```python
from build123d import *

# Parameters (mm, degrees)
SKETCH1_W               = 101.6
SKETCH1_H               = 203.2
BOSS_EXTRUDE1_DEPTH     = 101.6
SKETCH2_W               = 12.7
SKETCH2_H               = 12.7
SKETCH2_W_2             = 12.648057186
CUT_EXTRUDE1_DEPTH      = 203.2
SKETCH3_W               = 4.23418
SKETCH3_H               = 63.5
SKETCH3_W_2             = 63.551942814
SKETCH3_H_2             = 4.23418
SKETCH3_W_3             = 4.181475186
SKETCH3_W_4             = 8.466582
SKETCH3_H_3             = 8.46582
SKETCH3_W_5             = 8.46582
CUT_EXTRUDE2_DEPTH      = 200.025
SKETCH4_W               = 101.6
SKETCH4_H               = 25.341987408
CUT_EXTRUDE3_DEPTH      = 101.6
F_1_2_13_TAPPED_HOLE2_D = 10.71626
SKETCH7_W               = 13.255770889
SKETCH7_H               = 13.293622463
SKETCH7_W_2             = 13.104364594
SKETCH7_H_2             = 13.217919315
CUT_EXTRUDE4_DEPTH      = 190.5


with BuildPart() as part:
    # Sketch1 → Boss-Extrude1 (new body)
    with BuildSketch(Plane(origin=(0, 0, 0), x_dir=(0, 0, -1), z_dir=(1, 0, 0))):
        Rectangle(SKETCH1_W, SKETCH1_H)
    extrude(amount=BOSS_EXTRUDE1_DEPTH)

    # Sketch2 → Cut-Extrude1 (cut)
    with BuildSketch(Plane(origin=(0, 101.6, 0), x_dir=(1, 0, 0), z_dir=(0, 1, 0))):
        with Locations((9.525, 41.275)):
            Rectangle(SKETCH2_W, SKETCH2_H)
        with Locations((9.525, -41.275)):
            Rectangle(SKETCH2_W, SKETCH2_H)
        with Locations((92.100971407, -41.275)):
            Rectangle(SKETCH2_W_2, SKETCH2_H)
        with Locations((92.100971407, 41.275)):
            Rectangle(SKETCH2_W_2, SKETCH2_H)
    extrude(amount=-CUT_EXTRUDE1_DEPTH, mode=Mode.SUBTRACT)

    # Sketch3 → Cut-Extrude2 (cut)
    with BuildSketch(Plane(origin=(0, 101.6, 0), x_dir=(1, 0, 0), z_dir=(0, 1, 0))):
        with Locations((16.93291, 0)):
            Rectangle(SKETCH3_W, SKETCH3_H)
        with Locations((50.825971407, 0)):
            Rectangle(SKETCH3_W_2, SKETCH3_H)
        with Locations((50.825971407, 33.86709)):
            Rectangle(SKETCH3_W_2, SKETCH3_H_2)
        with Locations((84.692680407, 0)):
            Rectangle(SKETCH3_W_3, SKETCH3_H)
        with Locations((94.191709, 0)):
            Rectangle(SKETCH3_W_4, SKETCH3_H)
        with Locations((50.825971407, 43.39209)):
            Rectangle(SKETCH3_W_2, SKETCH3_H_3)
        with Locations((7.40791, 0)):
            Rectangle(SKETCH3_W_5, SKETCH3_H)
        with Locations((50.825971407, -43.39209)):
            Rectangle(SKETCH3_W_2, SKETCH3_H_3)
        with Locations((50.825971407, -33.86709)):
            Rectangle(SKETCH3_W_2, SKETCH3_H_2)
    extrude(amount=-CUT_EXTRUDE2_DEPTH, mode=Mode.SUBTRACT)

    # Sketch4 → Cut-Extrude3 (cut)
    with BuildSketch(Plane(origin=(101.6, 0, 0), x_dir=(0, 0, -1), z_dir=(1, 0, 0))):
        with Locations((0, 88.929006296)):
            Rectangle(SKETCH4_W, SKETCH4_H)
    extrude(amount=-CUT_EXTRUDE3_DEPTH, mode=Mode.SUBTRACT)

    # 1/2-13 Tapped Hole2 (through all)
    with Locations(Plane(origin=(50.825971407, -98.425, 0), x_dir=(0, 0, 1), z_dir=(0, 1, 0))):
        with Locations((0, 0)):
            Hole(F_1_2_13_TAPPED_HOLE2_D / 2)

    # Sketch7 → Cut-Extrude4 (cut)
    with BuildSketch(Plane(origin=(0, 76.258012592, 0), x_dir=(1, 0, 0), z_dir=(0, 1, 0))):
        with Locations((9.802885445, 40.978188769)):
            Rectangle(SKETCH7_W, SKETCH7_H)
        with Locations((91.872817703, 40.978188769)):
            Rectangle(SKETCH7_W_2, SKETCH7_H)
        with Locations((91.872817703, -41.016040343)):
            Rectangle(SKETCH7_W_2, SKETCH7_H_2)
        with Locations((9.802885445, -41.016040343)):
            Rectangle(SKETCH7_W, SKETCH7_H_2)
    extrude(amount=-CUT_EXTRUDE4_DEPTH, mode=Mode.SUBTRACT)


solid = part.part
```
Build history of the part. All positions in model axes, mm. A direction names the side the tool comes from. Round coordinates to 2 decimals unless told otherwise and drop trailing zeros. Order: outer loops, then holes, each group sorted by start corner. A loop starts at its lowest first (then second) coordinate and runs counter-clockwise, first axis right, second up. Notation, with made-up numbers: (30, -34) -> (83, -34) arc R18 ccw to (83, -2) -> close; hole circle Ø10 at (-11.75, 37.25). An arc over 180 degrees is marked (long way). Answer in a Markdown table with one row per item.
1) Wall check: L1, parallel to X at y = 38.5, z = 0 (3 decimals); L2, parallel to Z at x = 23, y = -46.5 (3 decimals); L3, parallel to Z at x = 83, y = -92.5. Give the ranges that are in metal, low to high.
Values:
| item | result |
|---|---|
| L1 | 0 to 3.175, 11.641 to 14.816, 86.783 to 89.958, 98.425 to 101.6 |
| L2 | -50.8 to -47.625, -39.159 to -35.984, 35.984 to 39.159, 47.625 to 50.8 |
| L3 | -50.8 to -31.75, 31.75 to 50.8 |
2) Band-saw the part on A-A on z = 44. Give the cut face in (x, y) (3 decimals).
Values:
| item | result |
|---|---|
| outline | (0, -101.6) -> (3.175, -101.6) -> (3.175, 76.258) -> (0, 76.258) -> close; (16.431, -101.6) -> (85.321, -101.6) -> (85.321, 76.258) -> (82.602, 76.258) -> (82.602, -98.425) -> (19.05, -98.425) -> (19.05, 76.258) -> (16.431, 76.258) -> close; (98.425, -101.6) -> (101.6, -101.6) -> (101.6, 76.258) -> (98.425, 76.258) -> close |
3) Which spindle directions (+Z, -Z, +X, -X, +Y, -Y) get a long thin tool onto all of the face, cutting with end or side? Do faces 3 (the flat face through (19.05, -10, -34)), 4 (the flat face through (3.175, -11, 41)), 5 (the flat face through (61, -101.6, 1)). Say none if no direction does.
Values:
| item | result |
|---|---|
| face 3 | +Y |
| face 4 | +Y, -Y |
| face 5 | +Z, -Z, +X, -X, -Y |
4) Band-saw the part on C-C on z = 0. Give the cut face in (x, y) (3 decimals), and give its area (3 significant figures).
Values:
| item | result |
|---|---|
| outline | (0, -101.6) -> (45.468, -101.6) -> (45.468, -98.425) -> (14.816, -98.425) -> (14.816, 76.258) -> (11.641, 76.258) -> (11.641, -98.425) -> (3.175, -98.425) -> (3.175, 76.258) -> (0, 76.258) -> close; (56.184, -101.6) -> (101.6, -101.6) -> (101.6, 76.258) -> (98.425, 76.258) -> (98.425, -98.425) -> (89.958, -98.425) -> (89.958, 76.258) -> (86.783, 76.258) -> (86.783, -98.425) -> (56.184, -98.425) -> close |
| area | 2,510 mm2 |
5) Mould opens along X. For faces 1 (the flat face through (50, -14, 50.8)), 2 (the flat face through (3.175, -10, 0)) say: released by +X, released by -X, zero draft, split by the parting line, or undercut.
Values:
| item | result |
|---|---|
| face 1 | zero draft |
| face 2 | undercut |
6) Pin check, flat tip, straight feed: P1, Ø2.5, axis at x = 60.5, z = 42.5, coming from the +Y side (3 decimals). Stop position of the tip, or through.
Values:
| item | result |
|---|---|
| P1 | y = -98.425 |
7) Band-saw the part on D-D on z = 27. Give the cut face in (x, y) (3 decimals), and give its area (3 significant figures).
Values:
| item | result |
|---|---|
| outline | (0, -101.6) -> (101.6, -101.6) -> (101.6, 76.258) -> (98.425, 76.258) -> (98.425, -98.425) -> (89.958, -98.425) -> (89.958, 76.258) -> (86.783, 76.258) -> (86.783, -98.425) -> (14.816, -98.425) -> (14.816, 76.258) -> (11.641, 76.258) -> (11.641, -98.425) -> (3.175, -98.425) -> (3.175, 76.258) -> (0, 76.258) -> close |
| area | 2,540 mm2 |
8) Band-saw the part on B-B on x = 42.5. Give the cut face in (y, z) (3 decimals), and give its area (3 significant figures).
Values:
| item | result |
|---|---|
| outline | (-101.6, -50.8) -> (76.258, -50.8) -> (76.258, -47.625) -> (-98.425, -47.625) -> (-98.425, -39.159) -> (76.258, -39.159) -> (76.258, -35.984) -> (-98.425, -35.984) -> (-98.425, 35.984) -> (76.258, 35.984) -> (76.258, 39.159) -> (-98.425, 39.159) -> (-98.425, 47.625) -> (76.258, 47.625) -> (76.258, 50.8) -> (-101.6, 50.8) -> close |
| area | 2,540 mm2 |
